Work out the finished part from the listing and answer in its coordinate system (mm). A direction names the side the tool comes from. Coordinates: 2 decimals unless noted, no trailing zeros. Order: outer loops, then holes, each group sorted by start corner. A loop starts at its lowest first (then second) coordinate and runs counter-clockwise, first axis right, second up. Notation, with made-up numbers: (-25, 63.5) -> (-19, 63.5) arc R27 cw to (-19, 95.5) -> close; hole circle Ø5 at (74.25, 53). An arc over 180 degrees is marked (long way). Use one line per item in the form item = value.
Autodesk Inventor part; units mm, degrees
ref_plane "YZ Plane" through (0, 0, 0) normal (1, 0, 0) x (0, 1, 0)
ref_plane "XZ Plane" through (0, 0, 0) normal (0, 1, 0) x (-1, 0, 0)
ref_plane "XY Plane" through (0, 0, 0) normal (0, 0, 1) x (1, 0, 0)
sketch "Sketch1" plane through (0, 0, 0) normal (0, 0, 1) x (1, 0, 0)
  line L0 (55.4, 13.1) -> (-55.4, 13.1)
  line L1 (-55.4, 13.1) -> (-55.4, -13.1)
  line L2 (-55.4, -13.1) -> (55.4, -13.1)
  line L3 (55.4, -13.1) -> (55.4, 13.1)
  line L4 (55.4, 13.1) -> (-55.4, -13.1) construction
  line L5 (-55.4, 13.1) -> (55.4, -13.1) construction
  point P0 (0, 0)
  dimension "d0" = 110.8
  dimension "d1" = 26.2
extrude "Extrusion1" add sketch "Sketch1" along normal blind 11
sketch "Sketch2" plane through (55.4, -13.1, 0) normal (1, 0, 0) x (0, 0, -1)
  line L0 (0, 0) -> (0, 26.2)
  line L1 (0, 26.2) -> (-11, 26.2)
  line L2 (-11, 0) -> (-11, 26.2)
  line L3 (0, 0) -> (-11, 0)
  line L4 (-11, 26.2) -> (-11, 0)
  line L5 (-11, 26.2) -> (-5, 26.2)
  line L6 (-5, 26.2) -> (-5, 23.2)
  line L7 (-5, 23.2) -> (-11, 23.2)
  line L8 (-11, 23.2) -> (-11, 26.2)
  line L9 (-11, 23.2) -> (-8, 23.2)
  line L10 (-8, 23.2) -> (-8, 20.2)
  line L11 (-8, 20.2) -> (-11, 20.2)
  line L12 (-11, 20.2) -> (-11, 23.2)
  line L13 (-11, 26.2) -> (-5, 26.2)
  line L14 (-5, 26.2) -> (-5, 10.2)
  line L15 (-5, 10.2) -> (-11, 10.2)
  line L16 (-11, 10.2) -> (-11, 26.2)
  line L17 (-11, 10.2) -> (-5, 10.2)
  line L18 (-5, 10.2) -> (-5, 13.2)
  line L19 (-5, 13.2) -> (-11, 13.2)
  line L20 (-11, 13.2) -> (-11, 10.2)
  line L21 (-11, 13.2) -> (-8, 13.2)
  line L22 (-8, 13.2) -> (-8, 16.2)
  line L23 (-8, 16.2) -> (-11, 16.2)
  line L24 (-11, 16.2) -> (-11, 13.2)
  point P0 (0, 13.1)
  point P1 (-11, 20.2)
  dimension "d4" = 6
  dimension "d5" = 3
  dimension "d6" = 3
  dimension "d7" = 3
  dimension "d8" = 16
  dimension "d9" = 3
  dimension "d10" = 3
  dimension "d11" = 3
extrude "Extrusion2" cut sketch "Sketch2" against normal blind 107.8 contours L14 L19 L22 L23 L2 L11 L10 L7
fillet "Fillet1" radius 2 5 edges at (55.4, 10.1, 11) (55.4, -5, 11) (-55.4, 0, 11) (55.4, 0, 0) (-55.4, 0, 0)
sketch "Sketch4" plane through (-53.4, -13.1, 0) normal (0, -1, 0) x (1, 0, 0)
  arc A0 (-2, 2) -> (0, 0) centre (0, 2) ccw
  line L0 (0, 0) -> (106.8, 0)
  arc A1 (106.8, 0) -> (108.8, 2) centre (106.8, 2) ccw
  line L1 (108.8, 2) -> (108.8, 9)
  arc A2 (108.8, 9) -> (106.8, 11) centre (106.8, 9) ccw
  line L2 (0, 11) -> (106.8, 11)
  arc A3 (0, 11) -> (-2, 9) centre (0, 9) ccw
  line L3 (-2, 2) -> (-2, 9)
  circle A4 centre (98.8, 5.5) radius 4.1
  circle A5 centre (91.8, 5.5) radius 2.15
  line L4 (91.8, 7.65) -> (95.3089, 7.65)
  line L5 (91.8, 3.35) -> (95.3089, 3.35)
  circle A6 centre (15, 5.5) radius 4.1
  circle A7 centre (8, 5.5) radius 2.15
  line L6 (8, 3.35) -> (11.5089, 3.35)
  line L7 (8, 7.65) -> (11.5089, 7.65)
  point P0 (53.4, 0)
  point P1 (108.8, 5.5)
  point P2 (12.2407, 8.5325)
  point P3 (8.4381, 3.3951)
  point P4 (11.1965, 3.9692)
  point P5 (-2, 5.5)
  dimension "d19" = 8.2
  dimension "d20" = 4.3
  dimension "d21" = 7
  dimension "d22" = 0
  dimension "d23" = 10
  dimension "d24" = 8.2
  dimension "d25" = 4.3
  dimension "d26" = 7
  dimension "d27" = 10
  dimension "d28" = 0
  dimension "d40" = 0
extrude "Extrusion4" cut sketch "Sketch4" against normal blind 5.2 contours A4 | A4 L5 A5 L4 | A5 | A6 | A6 L6 A7 L7 | A7
sketch "Sketch5" plane through (-53.4, -13.1, 0) normal (0, -1, 0) x (1, 0, 0)
  arc A0 (8, 7.65) -> (8, 3.35) centre (8, 5.5) ccw
  arc A1 (11.5089, 3.35) -> (11.5089, 7.65) centre (15, 5.5) ccw
  arc A2 (91.8, 7.65) -> (91.8, 3.35) centre (91.8, 5.5) ccw
  line L0 (91.8, 7.65) -> (95.3089, 7.65)
  arc A3 (95.3089, 3.35) -> (95.3089, 7.65) centre (98.8, 5.5) ccw
  line L1 (95.3089, 3.35) -> (91.8, 3.35)
  arc A4 (-2, 2) -> (0, 0) centre (0, 2) ccw
  line L2 (0, 0) -> (106.8, 0)
  arc A5 (106.8, 0) -> (108.8, 2) centre (106.8, 2) ccw
  line L3 (108.8, 2) -> (108.8, 9)
  arc A6 (108.8, 9) -> (106.8, 11) centre (106.8, 9) ccw
  line L4 (0, 11) -> (106.8, 11)
  arc A7 (0, 11) -> (-2, 9) centre (0, 9) ccw
  line L5 (-2, 2) -> (-2, 9)
  circle A8 centre (8, 5.5) radius 4.1
  line L6 (8, 9.6) -> (15, 9.6)
  line L7 (8, 1.4) -> (15, 1.4)
  arc A9 (11.5089, 3.35) -> (11.5089, 7.65) centre (15, 5.5) ccw
  circle A10 centre (91.8, 5.5) radius 4.1
  line L8 (91.8, 9.6) -> (98.8, 9.6)
  line L9 (98.8, 1.4) -> (91.8, 1.4)
  line L10 (8, 7.65) -> (11.5089, 7.65)
  line L11 (11.5089, 3.35) -> (8, 3.35)
  arc A11 (8, 7.65) -> (8, 3.35) centre (8, 5.5) ccw
  point P0 (53.4, 0)
  point P1 (19.1, 5.5)
  point P2 (19.1, 5.5)
  point P3 (5.85, 5.5)
  point P4 (89.65, 5.5)
  point P5 (12.4867, 2.2607)
  point P6 (12.4867, 8.7393)
  point P7 (96.275, 2.2698)
  point P8 (96.275, 8.7302)
  point P9 (5.85, 5.5)
  point P10 (95.2911, 7.65)
  point P11 (95.2911, 3.35)
  point P12 (11.4911, 3.35)
  point P13 (11.4911, 7.65)
  dimension "d32" = 8.2
  dimension "d33" = 0
  dimension "d35" = 8.2
  dimension "d36" = 0
  dimension "d42" = 0
  dimension "d43" = 0
extrude "Extrusion5" cut sketch "Sketch5" along normal blind 3.2 from surface at -5.2 contours L10 A8 L11 A0 | A0 L11 A8 L10 | A8 L6 A1 L10 | L11 A1 L7 A8 | L0 A10 L1 A2 | A2 L1 A10 L0 | A10 L8 A3 L0 | L1 A3 L9 A10
properties part number "module-slot" material "PC/ABS Plastic"
(1) The mould has two halves that part along X. Classify faces 5 (the cylindrical face through (49.5, -11.1, 5.4)), 6 (the flat face through (2, 5, 5)), 7 (the cylindrical face through (34.3, -9.5, 5.4)), 8 (the flat face through (55.4, -0.2, 5.5)): released by +X, released by -X, zero draft, split by the parting line, or undercut.
Data:
face_5 = undercut
face_6 = zero draft
face_7 = undercut
face_8 = released by +X
(2) Straight lines are drawn through the part: line 1 along X through (y, z) = (-10.3, 5.5); line 2 along X through (y, z) = (-11.7, 5.5); line 3 along Y through (x, z) = (-25, 6). For each, find the intervals that lie inside material, in ascending order.
Data:
line_1 = -55.4 to -49.5, -34.3 to 34.3, 49.5 to 55.4
line_2 = -55.4 to -47.55, -34.3 to 36.25, 49.5 to 55.4
line_3 = -13.1 to 0.1, 10.1 to 13.1
(3) Each of these flat-tipped pins is pushed along its axis until it touches: P1, Ø2.5, axis at x = -39, z = 7, coming from the -Y side; P2, Ø3, axis at x = -2, y = 5.5, coming from the +Z side. Where does it stop, or does it pass through?
Data:
P1 = -7.9
P2 = 5
(4) Which of the six approach directions +Z, -Z, +X, -X, +Y, -Y give full straight-line access (tool end or side, diameter ignored) to faces 1 (the flat face through (-1, 0, 0)), 2 (the flat face through (40, -12, 7.65)), 3 (the flat face through (-42, -7.9, 6)), 4 (the flat face through (2, 0.1, 6))?
Data:
face_1 = -Z, +X, -X, +Y, -Y
face_2 = -Y
face_3 = none
face_4 = +X
(5) Section A-A on x = 0 is taken. Write down the section's boundary in (y, z).
Data:
outline = (-13.1, 0) -> (13.1, 0) -> (13.1, 11) -> (7.1, 11) -> (7.1, 8) -> (10.1, 8) -> (10.1, 5) -> (0.1, 5) -> (0.1, 8) -> (3.1, 8) -> (3.1, 11) -> (-13.1, 11) -> close
